For this review, take the finished solid that the model builds, in its own axes (mm). A direction names the side the tool comes from. Round coordinates to 2 decimals unless told otherwise and drop trailing zeros. Order: outer loops, then holes, each group sorted by start corner. A loop starts at its lowest first (then second) coordinate and runs counter-clockwise, first axis right, second up. Notation, with made-up numbers: (19, -20.75) - (35, -20.75) arc R36 ccw to (35, 15.25) - close; hole circle Ø3 at (-13, -2). An arc over 180 degrees is marked (long way). One line per item, written item: value.
```python
from build123d import *

# Parameters (mm, degrees)
ESQUISSE1_W              = 112.172532808
ESQUISSE1_H              = 92.061088164
BOSS_EXTRU_1_DEPTH       = 98
ESQUISSE2_W              = 63.4
ESQUISSE2_H              = 27.4
ENL_V_MAT_EXTRU_1_DEPTH  = 122.93637795
ENL_V_MAT_EXTRU_2_DEPTH  = 122.93637795
ESQUISSE8_R              = 1.2
ENL_V_MAT_EXTRU_5_DEPTH  = 122.93637795
ENL_V_MAT_EXTRU_10_DEPTH = 36
BOSS_EXTRU_2_DEPTH       = 98
ESQUISSE15_R             = 0.9
ENL_V_MAT_EXTRU_11_DEPTH = 5
ENL_V_MAT_EXTRU_13_DEPTH = 33
ESQUISSE18_R             = 10
ENL_V_MAT_EXTRU_14_DEPTH = 7
ESQUISSE19_W             = 80.9
ESQUISSE19_H             = 35.571792003
ENL_V_MAT_EXTRU_15_DEPTH = 119.955890106
BOSS_EXTRU_3_DEPTH       = 2
ESQUISSE22_R             = 1.2
ENL_V_MAT_EXTRU_16_DEPTH = 14


with BuildPart() as part:
    # Esquisse1 → Boss.-Extru.1 (new body)
    with BuildSketch(Plane.XY):
        Rectangle(ESQUISSE1_W, ESQUISSE1_H)
    extrude(amount=BOSS_EXTRU_1_DEPTH)

    # Esquisse2 → Enlèv. mat.-Extru.1 (cut, through all)
    with BuildSketch(Plane.XY.offset(98)):
        with Locations((0, 30.491247921)):
            Rectangle(ESQUISSE2_W, ESQUISSE2_H)
    extrude(amount=-ENL_V_MAT_EXTRU_1_DEPTH, mode=Mode.SUBTRACT)

    # Esquisse3 → Enlèv. mat.-Extru.2 (cut, through all)
    with BuildSketch(Plane.XY.offset(98)):
        with BuildLine():
            Line((-29.4, 14.791247921), (29.4, 14.791247921))
            ThreePointArc((29.4, 14.791247921), (40.8, 3.391247921), (29.4, -8.008752079))
            Line((29.4, -8.008752079), (-29.4, -8.008752079))
            ThreePointArc((-29.4, -8.008752079), (-40.8, 3.391247921), (-29.4, 14.791247921))
        make_face()
    extrude(amount=-ENL_V_MAT_EXTRU_2_DEPTH, mode=Mode.SUBTRACT)

    # Esquisse8 → Enlèv. mat.-Extru.5 (cut, through all)
    with BuildSketch(Plane(origin=(0, 0, 0), x_dir=(-1, 0, 0), z_dir=(0, 0, -1))):
        with Locations((36.342435472, 16.729092577)):
            Circle(ESQUISSE8_R)
        with Locations(Location((-36.342435472, 16.729092577, 0), (0, 0, 180))):
            Circle(ESQUISSE8_R)
        Polygon((40.45, -46.030544082), (40.45, -10.458752079), (43.831541667, 3.591247921), (40.45, 20.287049631), (34.90419829, 20.287049631), (34.90419829, 46.030544082), (56.086266404, 46.030544082), (56.086266404, -46.030544082), align=None)
        Polygon((-40.45, -46.030544082), (-40.45, -10.458752079), (-43.831541667, 3.591247921), (-40.45, 20.287049631), (-35.235952742, 46.030544082), (-56.086266404, 46.030544082), (-56.086266404, -46.030544082), align=None)
    extrude(amount=-ENL_V_MAT_EXTRU_5_DEPTH, mode=Mode.SUBTRACT)

    # Esquisse13 → Enlèv. mat.-Extru.10 (cut)
    with BuildSketch(Plane(origin=(0, 46.030544082, 0), x_dir=(1, 0, 0), z_dir=(0, 1, 0))):
        with BuildLine():
            Line((29.401511347, -13.631097944), (29.401511347, -78.444504203))
            ThreePointArc((29.401511347, -78.444504203), (20.430009822, -87.416005728), (11.458508297, -78.444504203))
            Line((11.458508297, -78.444504203), (11.458508297, -13.631097944))
            ThreePointArc((11.458508297, -13.631097944), (20.430009822, -4.659596419), (29.401511347, -13.631097944))
        make_face()
    extrude(amount=-ENL_V_MAT_EXTRU_10_DEPTH, mode=Mode.SUBTRACT)

    # Esquisse14 → Boss.-Extru.2 (add, through all)
    with BuildSketch(Plane(origin=(0, 0, 0), x_dir=(-1, 0, 0), z_dir=(0, 0, -1))):
        Polygon((-35.235952742, 46.030544082), (-34.181307811, 51.237678691), (-29.786849485, 51.237678691), (-29.786849485, 46.030544082), align=None)
    extrude(amount=-BOSS_EXTRU_2_DEPTH)

    # Esquisse15 → Enlèv. mat.-Extru.11 (cut)
    with BuildSketch(Plane(origin=(42.803048455, 8.669262748, 0), x_dir=(0, 0, -1), z_dir=(0.980099310455717, 0.19850778736419453, 0))):
        with Locations(Location((-5.012556966, -1.831122741, 0), (0, 0, 90))):
            Circle(ESQUISSE15_R)
        with Locations(Location((-5.012556966, 38.868877259, 0), (0, 0, 90))):
            Circle(ESQUISSE15_R)
        with Locations(Location((-93.012556966, -1.831122741, 0), (0, 0, 90))):
            Circle(ESQUISSE15_R)
        with Locations(Location((-93.012556966, 38.868877259, 0), (0, 0, 90))):
            Circle(ESQUISSE15_R)
    extrude(amount=-ENL_V_MAT_EXTRU_11_DEPTH, mode=Mode.SUBTRACT)

    # Esquisse17 → Enlèv. mat.-Extru.13 (cut)
    with BuildSketch(Plane.ZY.offset(34.90419829)):
        with BuildLine():
            Line((11.891222977, 39.441182616), (75.540539517, 39.441182616))
            ThreePointArc((75.540539517, 39.441182616), (85.11760601, 29.864116124), (75.540539517, 20.287049631))
            Line((75.540539517, 20.287049631), (11.891222977, 20.287049631))
            ThreePointArc((11.891222977, 20.287049631), (2.314156484, 29.864116124), (11.891222977, 39.441182616))
        make_face()
    extrude(amount=-ENL_V_MAT_EXTRU_13_DEPTH, mode=Mode.SUBTRACT)

    # Esquisse18 → Enlèv. mat.-Extru.14 (cut)
    with BuildSketch(Plane(origin=(40.614547147, -9.775073555, 0), x_dir=(0, 0, -1), z_dir=(0.9722372677043548, -0.23399721213461214, 0))):
        with Locations(Location((-81, 13.74800362, 0), (0, 0, 32.947816907))):
            Circle(ESQUISSE18_R)
    extrude(amount=-ENL_V_MAT_EXTRU_14_DEPTH, mode=Mode.SUBTRACT)

    # Esquisse19 → Enlèv. mat.-Extru.15 (cut, through all)
    with BuildSketch(Plane(origin=(0, 0, 0), x_dir=(-1, 0, 0), z_dir=(0, 0, -1))):
        with Locations((0, -28.244648081)):
            Rectangle(ESQUISSE19_W, ESQUISSE19_H)
    extrude(amount=-ENL_V_MAT_EXTRU_15_DEPTH, mode=Mode.SUBTRACT)

    # Esquisse21 → Boss.-Extru.3 (add)
    with BuildSketch(Plane.XZ.offset(10.458752079)):
        Polygon((-40.45, 98), (40.45, 98), (66, 98), (66, 0), (40.45, 0), (-40.45, 0), (-66, 0), (-66, 98), align=None)
    extrude(amount=-BOSS_EXTRU_3_DEPTH)

    # Esquisse22 → Enlèv. mat.-Extru.16 (cut)
    with BuildSketch(Plane.XZ.offset(10.458752079)):
        with Locations(Location((43.537561985, 90.712580413, 0), (0, 0, 270))):
            Circle(ESQUISSE22_R)
        with Locations(Location((55, 91.492580413, 0), (0, 0, 270))):
            Circle(ESQUISSE22_R)
        with Locations(Location((37.317561985, 42.512580413, 0), (0, 0, 270))):
            Circle(ESQUISSE22_R)
        with Locations(Location((55, 41.492580413, 0), (0, 0, 270))):
            Circle(ESQUISSE22_R)
        with Locations(Location((-55, 41.492580413, 0), (0, 0, 270))):
            Circle(ESQUISSE22_R)
        with Locations(Location((-37.922438015, 42.512580413, 0), (0, 0, 270))):
            Circle(ESQUISSE22_R)
        with Locations(Location((-55, 91.492580413, 0), (0, 0, 270))):
            Circle(ESQUISSE22_R)
        with Locations(Location((-39.065455989, 90.712580413, 0), (0, 0, 270))):
            Circle(ESQUISSE22_R)
    extrude(amount=-ENL_V_MAT_EXTRU_16_DEPTH, mode=Mode.SUBTRACT)


solid = part.part
```
Item 1: Wall thickness on line 1 (Y direction, x = -20, z = 50.5); line 2 (Y direction, x = 31, z = 13); line 3 (Y direction, x = 49.5, z = 55.5): over which ranges is each line inside the solid? List them lowest first.
Returned:
line 1: -10.46 to -8.01, 14.79 to 16.79, 44.19 to 46.03
line 2: -10.46 to -7.9, 14.68 to 16.79, 44.19 to 51.24
line 3: -10.46 to -8.46
Item 2: Take a section at C-C (z = 24). Count the separate pieces of the cut face and the enclosed holes in it, plus the area to 3 significant figures.
Returned:
separate pieces: 2
enclosed holes: 2
area: 966 mm^2
Item 3: The part is to be moulded in two halves that separate along Y. For faces 5 (the flat face through (0, 16, 98)), 6 (the flat face through (38.8, 12.6, 80.6)), 7 (the flat face through (1, -10.459, 50)), say which applies: +Y half, -Y half, draft (parallel to the pull), parting line (faces both ways), or undercut.
Returned:
face 5: draft
face 6: undercut
face 7: -Y half
Item 4: Take a section at B-B (y = 41). Write out the cut boundary in (x, z).
Returned:
outline: (-34.9, 0) - (-31.7, 0) - (-31.7, 98) - (-34.9, 98) - close; (31.7, 0) - (36.25, 0) - (36.25, 98) - (31.7, 98) - close
Item 5: Machinability: for faces 1 (the cylindrical face through (-33.325, 30.075, 85.115)), 2 (the cylindrical face through (20.23, 45.12, 4.66)), 3 (the flat face through (-42.36, -2.52, 48.31)), 4 (the cylindrical face through (40.8, 3.6, 49.7)), which of the approach directions +Z, -Z, +X, -X, +Y, -Y give a long, thin tool a straight path to every point of the face, cutting with its end or side? Answer none if there is none.
Returned:
face 1: -X
face 2: +Y
face 3: +Z, -Z, -X
face 4: +Z, -Z
Item 6: Take a section at A-A (x = -25). Write out the cut boundary in (y, z), plus the area to 3 significant figures.
Returned:
outline: (-10.46, 0) - (-8.01, 0) - (-8.01, 98) - (-10.46, 98) - close; (14.79, 0) - (16.79, 0) - (16.79, 98) - (14.79, 98) - close; (44.19, 0) - (46.03, 0) - (46.03, 98) - (44.19, 98) - close
area: 616 mm^2
Item 7: For P1, Ø12.5, axis at x = -58, z = 71.5, coming from the +Y side; P2, Ø20.5, axis at y = 27, z = 44.5, coming from the -X side; P3, Ø7, axis at x = -34.5, z = 54, coming from the +Y side, all flat-tipped, find the tip position at first contact; note any pin that passes through.
Returned:
P1: y = -8.46
P2: x = -41.17
P3: y = 46.03
